Job drawing, mm, ordinate dimensions from the low corner. One solid piece. A direction names the side the tool comes from. Round coordinates to 2 decimals unless told otherwise and drop trailing zeros. Order: outer loops, then holes, each group sorted by start corner. A loop starts at its lowest first (then second) coordinate and runs counter-clockwise, first axis right, second up. Notation, with made-up numbers: (-23, 7.25) -> (14, 7.25) arc R18 cw to (14, 17.25) -> close; hole circle Ø3 at (25, -38). An arc over 180 degrees is marked (long way). Use CSV: the item, a comma, the result in double quotes.
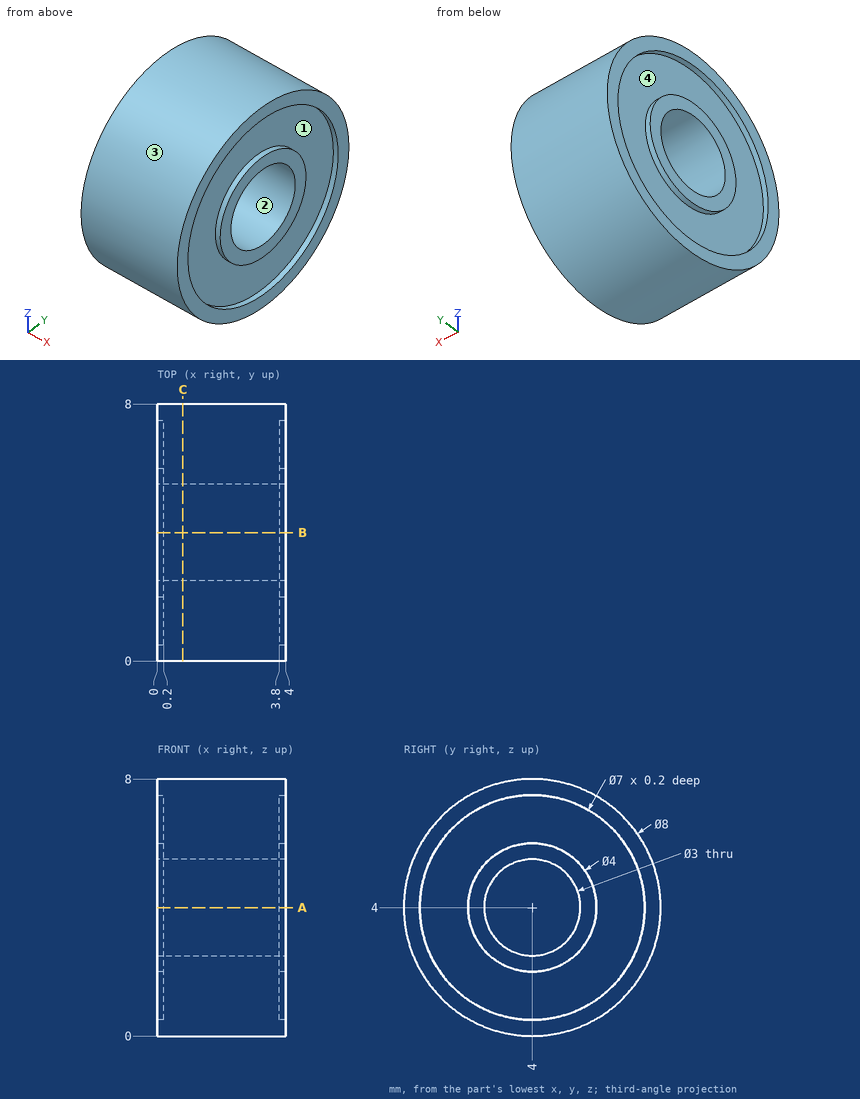
(1) Cut at C-C, the plane x = 0.8. Give the cut face in (y, z), then the cut area to 3 significant figures.
Reply:
outline,"circle Ø8 at (4, 4); hole circle Ø3 at (4, 4)"
area,"43.2 mm2"
(2) Drop a flat-ended pin along its axis: P1, Ø1, axis at x = 0.5, y = 2, coming from the -Z side. Give the stop position or say it passes through.
Reply:
P1,"z = 0.29"
(3) Pull direction Y, two halves, no side cores. Call the marked faces 3 and 4: released by +Y, released by -Y, zero draft, split by the parting line, or undercut.
Reply:
face 3,"split by the parting line"
face 4,"undercut"
(4) Which spindle directions (+Z, -Z, +X, -X, +Y, -Y) get a long thin tool onto all of the face, cutting with end or side? Do the marked faces 1 and 2. Say none if no direction does.
Reply:
face 1,"+X"
face 2,"+X, -X"
(5) Probe probe 1 along Y at (x, z) = (0.1, 4); probe 2 along Y at (x, z) = (1.45, 4); probe 3 along Y at (x, z) = (2.9, 5). List the from-to ranges inside material, lowest first. Write a range as [from, to].
Reply:
probe 1,"[0, 0.5], [2, 2.5], [5.5, 6], [7.5, 8]"
probe 2,"[0, 2.5], [5.5, 8]"
probe 3,"[0.13, 2.88], [5.12, 7.87]"
(6) Cut at A-A, the plane z = 4. Give the cut face in (x, y), then the cut area to 3 significant figures.
Reply:
outline,"(0, 0) -> (4, 0) -> (4, 0.5) -> (3.8, 0.5) -> (3.8, 2) -> (4, 2) -> (4, 2.5) -> (0, 2.5) -> (0, 2) -> (0.2, 2) -> (0.2, 0.5) -> (0, 0.5) -> close; (0, 5.5) -> (4, 5.5) -> (4, 6) -> (3.8, 6) -> (3.8, 7.5) -> (4, 7.5) -> (4, 8) -> (0, 8) -> (0, 7.5) -> (0.2, 7.5) -> (0.2, 6) -> (0, 6) -> close"
area,"18.8 mm2"
